For this review, take the finished solid that the model builds, in its own axes (mm). Face numbers are marked on the shaded views. A direction names the side the tool comes from. Round coordinates to 2 decimals unless told otherwise and drop trailing zeros. Order: outer loops, then holes, each group sorted by start corner. A loop starts at its lowest first (then second) coordinate and runs counter-clockwise, first axis right, second up.
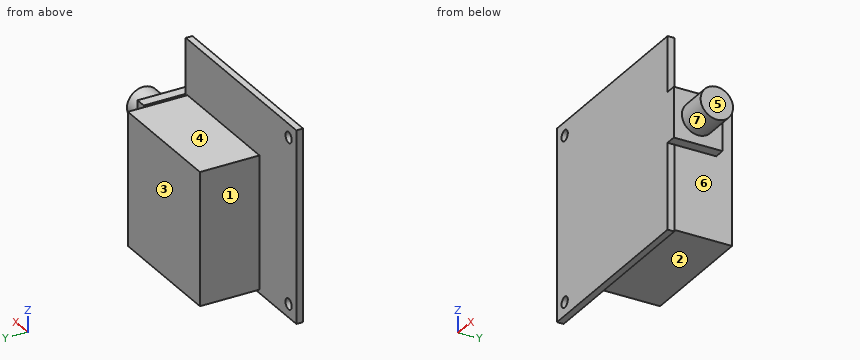
from build123d import *

# Parameters (mm, degrees)
SKETCH1_W           = 45
SKETCH1_H           = 45
SKETCH1_R           = 1.27
BOSS_EXTRUDE1_DEPTH = 1.5748
SKETCH2_W           = 29.307993044
SKETCH2_H           = 31.185373382
BOSS_EXTRUDE2_DEPTH = 14
SKETCH3_W           = 11.809383556
SKETCH3_H           = 11.428065242
BOSS_EXTRUDE3_DEPTH = 2.54
SKETCH4_R           = 3.81
BOSS_EXTRUDE4_DEPTH = 7.62


with BuildPart() as part:
    # Sketch1 → Boss-Extrude1 (new body)
    with BuildSketch(Plane(origin=(0, 0, 0), x_dir=(1, 0, 0), z_dir=(0, 1, 0))):
        Rectangle(SKETCH1_W, SKETCH1_H)
        with Locations(Location((-19.3504, 19.3504, 0), (0, 0, 270))):
            Circle(SKETCH1_R, mode=Mode.SUBTRACT)
        with Locations(Location((-19.3504, -19.3504, 0), (0, 0, 270))):
            Circle(SKETCH1_R, mode=Mode.SUBTRACT)
    extrude(amount=BOSS_EXTRUDE1_DEPTH)

    # Sketch2 → Boss-Extrude2 (add)
    with BuildSketch(Plane(origin=(0, 1.5748, 0), x_dir=(1, 0, 0), z_dir=(0, 1, 0))):
        with Locations((7.144475173, 6.07541137)):
            Rectangle(SKETCH2_W, SKETCH2_H)
    extrude(amount=BOSS_EXTRUDE2_DEPTH)

    # Sketch3 → Boss-Extrude3 (add)
    with BuildSketch(Plane(origin=(22.5, 0, 0), x_dir=(0, 0, -1), z_dir=(1, 0, 0))):
        with Locations((-3.598382338, 5.714032621)):
            Rectangle(SKETCH3_W, SKETCH3_H)
    extrude(amount=BOSS_EXTRUDE3_DEPTH)

    # Sketch4 → Boss-Extrude4 (add)
    with BuildSketch(Plane(origin=(25.04, 0, 0), x_dir=(0, 0, -1), z_dir=(1, 0, 0))):
        with Locations(Location((-3.598382338, 5.714032621, 0), (0, 0, 180))):
            Circle(SKETCH4_R)
    extrude(amount=BOSS_EXTRUDE4_DEPTH)


solid = part.part
(1) Tool access review of the marked faces 1, 2, 3 and 4: name each direction out of +Z, -Z, +X, -X, +Y, -Y from which nothing blocks a thin tool from reaching the whole face with its end or side.
(2) Add section C-C on z = -8.5. Give the boundary of the cut face in (x, y).
(3) Clearance check with flat-ended pins moving along their axes: P1, Ø0.8, axis at y = 0.5, z = 16, coming from the +X side; P2, Ø8, axis at y = 11.5, z = 14, coming from the +X side; P3, Ø5, axis at y = 6.5, z = 2.5, coming from the -X side; P4, Ø8, axis at x = -16.5, z = 4.5, coming from the +Y side. State where each tip first meets the part, or that it passes through.
(4) Add section A-A on y = 10.75. Give the boundary of the cut face in (x, z).
(5) Wall thickness on L1, parallel to Z at x = 24, y = 2; L2, parallel to Z at x = 15, y = 8.75; L3, parallel to X at y = 2.5, z = -8.5: over which ranges is each line inside the solid? List them lowest first.
(6) Add section D-D on y = 7.75. Give the boundary of the cut face in (x, z).
(7) Draft analysis for pull direction X (two halves, no side actions). For the marked faces 5, 6 and 7, state which applies: pulls with the +X half, pulls with the -X half, needs draft (parallel to the pull), parting line crosses it, or undercut.
(8) Add section B-B on x = 8. Give the boundary of the cut face in (y, z), plus the area to 3 significant figures.
Here are the results:
1. face 1: +Z, -Z, -X, +Y
1. face 2: -Z, +X, -X, +Y
1. face 3: +Z, -Z, +X, -X, +Y
1. face 4: +Z, +X, -X, +Y
2. outline: (-22.5, 0) - (22.5, 0) - (22.5, 1.57) - (21.8, 1.57) - (21.8, 15.57) - (-7.51, 15.57) - (-7.51, 1.57) - (-22.5, 1.57) - close
3. P1: stops at x = 22.5
3. P2: passes through
3. P3: stops at x = -7.51
3. P4: stops at y = 1.57
4. outline: (-7.51, -21.67) - (21.8, -21.67) - (21.8, 9.52) - (-7.51, 9.52) - close; (22.5, -2.31) - (25.04, -2.31) - (25.04, 9.5) - (22.5, 9.5) - close
5. L1: z = -2.31 to 9.5
5. L2: z = -21.67 to 9.52
5. L3: x = -7.51 to 21.8
6. outline: (-7.51, -21.67) - (21.8, -21.67) - (21.8, 9.52) - (-7.51, 9.52) - close; (22.5, -2.31) - (25.04, -2.31) - (25.04, 0.38) - (32.66, 0.38) - (32.66, 6.82) - (25.04, 6.82) - (25.04, 9.5) - (22.5, 9.5) - close
7. face 5: pulls with the +X half
7. face 6: undercut
7. face 7: needs draft
8. outline: (0, -22.5) - (1.57, -22.5) - (1.57, -21.67) - (15.57, -21.67) - (15.57, 9.52) - (1.57, 9.52) - (1.57, 22.5) - (0, 22.5) - close
8. area: 507 mm2
